```python
from build123d import *

# Parameters (mm, degrees)
BOSS_EXTRUDE1_DEPTH = 5
SKETCH2_R           = 5
SKETCH2_R_2         = 2.5
CUT_EXTRUDE1_DEPTH  = 10


with BuildPart() as part:
    # Sketch1 → Boss-Extrude1 (new body)
    with BuildSketch(Plane(origin=(0, 0, 0), x_dir=(1, 0, 0), z_dir=(0, 1, 0))):
        with BuildLine():
            Line((-175, 48), (175, 48))
            ThreePointArc((175, 48), (223, 0), (175, -48))
            Line((175, -48), (-175, -48))
            ThreePointArc((-175, -48), (-223, 0), (-175, 48))
        make_face()
    extrude(amount=BOSS_EXTRUDE1_DEPTH)

    # Sketch2 → Cut-Extrude1 (cut)
    with BuildSketch(Plane.XZ):
        with Locations(Location((175, 0, 0), (0, 0, 270))):
            Circle(SKETCH2_R)
        with Locations(Location((175, 18.65, 0), (0, 0, 270))):
            Circle(SKETCH2_R_2)
        with Locations(Location((175, -18.65, 0), (0, 0, 270))):
            Circle(SKETCH2_R_2)
        with Locations(Location((-175, -18.65, 0), (0, 0, 90))):
            Circle(SKETCH2_R_2)
        with Locations(Location((-175, 18.65, 0), (0, 0, 90))):
            Circle(SKETCH2_R_2)
        with Locations(Location((-175, 0, 0), (0, 0, 90))):
            Circle(SKETCH2_R)
    extrude(amount=-CUT_EXTRUDE1_DEPTH, mode=Mode.SUBTRACT)


solid = part.part
```
Check sheet for the modelled part. Datum: model origin and axes. Units: mm. Round coordinates to 2 decimals unless told otherwise and drop trailing zeros. Loops run counter-clockwise (first coordinate to the right, second up) from the corner with the lowest first, then second, coordinate; pieces in that order, holes last. Notation, with made-up numbers: (85.25, 83.5) - (119.25, 83.5) arc R22 ccw to (119.25, 103.5) - close; hole circle Ø2 at (37.25, 54). An arc over 180 degrees is marked (long way). Write item = value, one per line. Start each with the question number.
Q1. Thickness scan on L1, parallel to Z at x = -175, y = 1.55; L2, parallel to X at y = 3.15, z = 0; L3, parallel to X at y = 1.75, z = -19.5. Record the ranges inside material, lowest first.
Q2. Release check for a two-part mould opening along Z. For faces 1 (the face through (222.99, 2.46, -1.06)), 2 (the face through (179.957, 2.465, 0.651)), 3 (the face through (3, 5, -1)) record: pulls with the +Z half, pulls with the -Z half, needs draft (parallel to the pull), parting line crosses it, or undercut.
Q3. Section check B-B (z = 0). Record the boundary of the cut face in (x, y).
Q4. Section check A-A (y = 2.95). Record the boundary of the cut face in (x, z), plus the area to 3 significant figures.
Q5. Depth check by flat-ended pin: P1, Ø2, axis at y = 2.5, z = 15, coming from the +X side; P2, Ø4.5, axis at x = -175, z = -18.65, coming from the -Y side; P3, Ø2, axis at y = 3.5, z = 23.5, coming from the +X side. Enter the tip coordinate at first touch or a pass-through.
Derived:
q1.L1 = -48 to -21.15, -16.15 to -5, 5 to 16.15, 21.15 to 48
q1.L2 = -223 to -180, -170 to 170, 180 to 223
q1.L3 = -218.86 to -177.35, -172.65 to 172.65, 177.35 to 218.86
q2.face_1 = parting line crosses it
q2.face_2 = undercut
q2.face_3 = needs draft
q3.outline = (-223, 0) - (-180, 0) - (-180, 5) - (-223, 5) - close; (-170, 0) - (170, 0) - (170, 5) - (-170, 5) - close; (180, 0) - (223, 0) - (223, 5) - (180, 5) - close
q4.outline = (-175, -48) - (175, -48) arc R48 ccw to (175, 48) - (-175, 48) arc R48 ccw to start; hole circle Ø10 at (-175, 0); hole circle Ø5 at (-175, -18.65); hole circle Ø5 at (-175, 18.65); hole circle Ø10 at (175, 0); hole circle Ø5 at (175, -18.65); hole circle Ø5 at (175, 18.65)
q4.area = 40,600 mm^2
q5.P1 = 220.91
q5.P2 = through
q5.P3 = 217.4
